Can you work these out from the model? Positions are in its coordinate system, mm. A direction names the side the tool comes from. Give positions to 0.01 mm unless a question says otherwise; leave off trailing zeros. Loops run counter-clockwise (first coordinate to the right, second up) from the corner with the lowest first, then second, coordinate; pieces in that order, holes last. Notation, with made-up numbers: (65.5, 28) -> (84.5, 28) arc R26 ccw to (84.5, 46) -> close; hole circle Ø9 at (39.5, 17.5). An arc over 180 degrees is marked (long way). Return JSON: item names as keys, results as strings. Group by question number.
Q1. Thinking about a two-plate mould opening in X: for faces 1 (the cylindrical face through (-18.13, 2.46, -2.74)), 2 (the cylindrical face through (-18.13, 25.86, -2.74)), 3 (the flat face through (-9.95, 14, -13)), 4 (the flat face through (5, 14, -15.056)), which applies, pulls with the +X half, pulls with the -X half, needs draft (parallel to the pull), parting line crosses it, or undercut?
Q2. Suppose I cut it at A-A, the plane y = 21.7. Please give me the cut outline in (x, z), and give its area (3 significant figures).
Q3. Will these pins go through, and if not, where does the flat tip stop? pin 1 (1.5 mm diameter, centred on y = 3.5, z = -4.5, fed in from -X); pin 2 (4 mm diameter, centred on x = -16.61, z = -0.76, fed in from -Y); pin 3 (4 mm diameter, centred on y = 16.5, z = -11.5, fed in from -X); pin 4 (12 mm diameter, centred on x = 12, y = 24.5, fed in from +Z).
Q4. I need wall thicknesses on line 1 along Y through (x, z) = (-10, -2.75); line 2 along Z through (x, y) = (13.5, 8.25); line 3 along X through (y, z) = (2.5, 1.5). Which ranges of each line are inside material? Lowest first, please. Write a range as [from, to].
Q5. Suppose I cut it at C-C, the plane z = -4.25. Please give me the cut outline in (x, y).
Q6. Suppose I cut it at B-B, the plane y = 14.2. Please give me the cut outline in (x, z).
Q7. Which directions (+Z, -Z, +X, -X, +Y, -Y) give clear straight access to the entire face, cutting with the end or side of a thin tool? Please do faces 5 (the flat face through (9, 14, -10.056)), 6 (the flat face through (-14.941, 2.465, -10.113)).
Q8. Suppose I cut it at D-D, the plane x = -1.5. Please give me the cut outline in (y, z), and give its area (3 significant figures).
```python
from build123d import *
from build123d.topology import SkipClean

# Parameters (mm, degrees)
SKETCH1_R           = 2.5
BOSS_EXTRUDE1_DEPTH = 5
SKETCH2_R           = 2
BOSS_EXTRUDE2_DEPTH = 5
CUT_EXTRUDE1_DEPTH  = 42.079586535
BOSS_EXTRUDE3_START = -5
SKETCH3_R           = 2.5
BOSS_EXTRUDE3_DEPTH = 5


with BuildPart() as part:
    # Sketch1 → Boss-Extrude1 (new body)
    with BuildSketch(Plane(origin=(0, 0, 0), x_dir=(1, 0, 0), z_dir=(0, 1, 0))):
        with BuildLine():
            Line((20.049610011, 15.055516278), (-9.950389989, 15.055516278))
            Line((-9.950389989, 15.055516278), (-20.072425289, 5.030348084))
            ThreePointArc((-20.072425289, 5.030348084), (-20.555517893, -3.078179001), (-12.436571265, -2.824613195))
            Line((-12.436571265, -2.824613195), (0.632983681, 10.055516278))
            Line((0.632983681, 10.055516278), (20.049610011, 10.055516278))
            Line((20.049610011, 10.055516278), (20.049610011, 15.055516278))
        make_face()
        with Locations(Location((-16.611816522, 0.755516278, 0), (0, 0, 270))):
            Circle(SKETCH1_R, mode=Mode.SUBTRACT)
    extrude(amount=BOSS_EXTRUDE1_DEPTH)

    # Sketch2 → Boss-Extrude2 (add)
    with BuildSketch(Plane(origin=(0, 0, -15.055516278), x_dir=(-1, 0, 0), z_dir=(0, 0, -1))):
        with BuildLine():
            Line((9.950389989, 5), (9.950389989, 23.4))
            Line((9.950389989, 23.4), (9.950389989, 28.4))
            Line((9.950389989, 28.4), (-20.049610011, 28.4))
            Line((-20.049610011, 28.4), (-20.049610011, 5))
            Line((-20.049610011, 5), (-6.103175386, 5))
            ThreePointArc((-6.103175386, 5), (-6.022458727, 8.447445385), (-3.049610011, 6.7))
            ThreePointArc((-3.049610011, 6.7), (-3.302164625, 5.727151284), (-3.996044635, 5))
            Line((-3.996044635, 5), (9.950389989, 5))
        make_face()
        with Locations((-12.549610011, 14.2)):
            Circle(SKETCH2_R, mode=Mode.SUBTRACT)
        with Locations((-5.049610011, 21.7)):
            Circle(SKETCH2_R, mode=Mode.SUBTRACT)
        with Locations((2.450389989, 14.2)):
            Circle(SKETCH2_R, mode=Mode.SUBTRACT)
    extrude(amount=-BOSS_EXTRUDE2_DEPTH)

    # Sketch2_3 → Cut-Extrude1 (cut, through all)
    with SkipClean():  # the faces are left unmerged after this step: merging them gives an invalid solid
        with BuildSketch(Plane(origin=(0, 0, -15.055516278), x_dir=(-1, 0, 0), z_dir=(0, 0, -1))):
            with BuildLine():
                Line((-6.103175386, 5), (-3.996044635, 5))
                ThreePointArc((-3.996044635, 5), (-3.302164625, 5.727151284), (-3.049610011, 6.7))
                ThreePointArc((-3.049610011, 6.7), (-6.022458727, 8.447445385), (-6.103175386, 5))
            make_face()
            with BuildLine():
                ThreePointArc((-6.103175386, 5), (-5.049610011, 4.7), (-3.996044635, 5))
                Line((-3.996044635, 5), (-6.103175386, 5))
            make_face()
        extrude(amount=-CUT_EXTRUDE1_DEPTH, mode=Mode.SUBTRACT)

    # Sketch3 → Boss-Extrude3 (add)
    with SkipClean():  # the faces are left unmerged after this step: merging them gives an invalid solid
        with BuildSketch(Plane(origin=(0, 28.4, 0), x_dir=(1, 0, 0), z_dir=(0, 1, 0)).offset(BOSS_EXTRUDE3_START)):
            with BuildLine():
                Line((-9.950389989, 10.055516278), (-9.950389989, 15.055516278))
                Line((-9.950389989, 15.055516278), (-20.072425289, 5.030348084))
                ThreePointArc((-20.072425289, 5.030348084), (-20.555517893, -3.078179001), (-12.436571265, -2.824613195))
                Line((-12.436571265, -2.824613195), (0.632983681, 10.055516278))
                Line((0.632983681, 10.055516278), (-9.950389989, 10.055516278))
            make_face()
            with Locations(Location((-16.611816522, 0.755516278, 0), (0, 0, 270))):
                Circle(SKETCH3_R, mode=Mode.SUBTRACT)
        extrude(amount=BOSS_EXTRUDE3_DEPTH)


solid = part.part
```
Ans:
{
 "1": {"face 1": "undercut", "face 2": "undercut", "face 3": "pulls with the -X half", "face 4": "needs draft"},
 "2": {"outline": "(-9.95, -15.06) -> (3.05, -15.06) -> (3.05, -10.06) -> (-9.95, -10.06) -> close; (7.05, -15.06) -> (20.05, -15.06) -> (20.05, -10.06) -> (7.05, -10.06) -> close", "area": "130 mm^2"},
 "3": {"pin 1": "stops at x = -21.23", "pin 2": "passes through", "pin 3": "stops at x = -9.95", "pin 4": "stops at z = -10.06"},
 "4": {"line 1": "y = [0, 5], [23.4, 28.4]", "line 2": "z = [-15.06, -10.06]", "line 3": "x = [-21.63, -17.69], [-15.53, -11.09]"},
 "5": {"outline": "(-20.86, 0) -> (-5.26, 0) -> (-5.26, 5) -> (-20.86, 5) -> close; (-20.86, 23.4) -> (-5.26, 23.4) -> (-5.26, 28.4) -> (-20.86, 28.4) -> close"},
 "6": {"outline": "(-9.95, -15.06) -> (-4.45, -15.06) -> (-4.45, -10.06) -> (-9.95, -10.06) -> close; (-0.45, -15.06) -> (10.55, -15.06) -> (10.55, -10.06) -> (-0.45, -10.06) -> close; (14.55, -15.06) -> (20.05, -15.06) -> (20.05, -10.06) -> (14.55, -10.06) -> close"},
 "7": {"face 5": "+Z, +X", "face 6": "-Z, -X, +Y, -Y"},
 "8": {"outline": "(0, -15.06) -> (12.44, -15.06) -> (12.44, -10.06) -> (5, -10.06) -> (5, -7.95) -> (0, -7.95) -> close; (15.96, -15.06) -> (28.4, -15.06) -> (28.4, -7.95) -> (23.4, -7.95) -> (23.4, -10.06) -> (15.96, -10.06) -> close", "area": "145 mm^2"}
}
